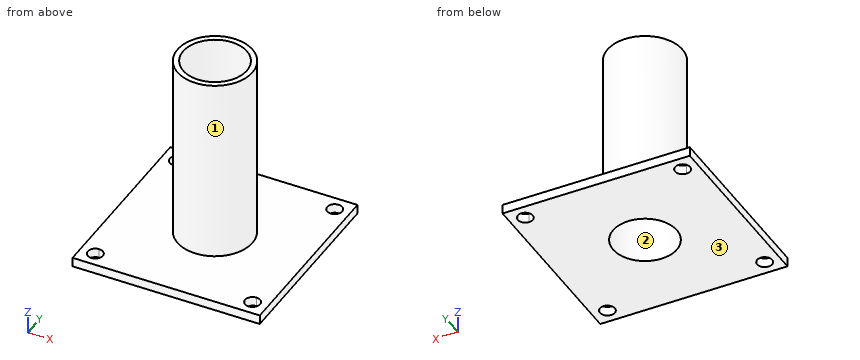
from build123d import *

# Parameters (mm, degrees)
F0_W     = 50
F0_H     = 50
F0_R     = 10
F0_R_2   = 8.5
F1_DEPTH = 2.5
F2_DEPTH = 25
F4_R     = 8.5
F4_R_2   = 2.5
F5_DEPTH = 2
F4_R_3   = 10
F6_DEPTH = 25
F7_R     = 2.5
F8_DEPTH = 25


with BuildPart() as f1:
    # F0 (on Top) → F1 (new body)
    with BuildSketch(Plane.XY):
        Rectangle(F0_W, F0_H)
        with BuildLine():
            ThreePointArc((-21, 19), (-22.414214, 22.414214), (-19, 21))
            Line((-19, 21), (19, 21))
            ThreePointArc((19, 21), (21, 23), (23, 21))
            ThreePointArc((23, 21), (22.414214, 19.585786), (21, 19))
            Line((21, 19), (21, -19))
            ThreePointArc((21, -19), (22.414214, -19.585786), (23, -21))
            ThreePointArc((23, -21), (21, -23), (19, -21))
            Line((19, -21), (-19, -21))
            ThreePointArc((-19, -21), (-22.414214, -22.414214), (-21, -19))
            Line((-21, -19), (-21, 19))
        make_face(mode=Mode.SUBTRACT)
        with BuildLine():
            Line((19, 21), (-19, 21))
            ThreePointArc((-19, 21), (-19.585786, 19.585786), (-21, 19))
            Line((-21, 19), (-21, -19))
            ThreePointArc((-21, -19), (-19.585786, -19.585786), (-19, -21))
            Line((-19, -21), (19, -21))
            ThreePointArc((19, -21), (19.585786, -19.585786), (21, -19))
            Line((21, -19), (21, 19))
            ThreePointArc((21, 19), (19.585786, 19.585786), (19, 21))
        make_face()
        Circle(F0_R, mode=Mode.SUBTRACT)
        Circle(F0_R)
        Circle(F0_R_2, mode=Mode.SUBTRACT)
    extrude(amount=-F1_DEPTH)

    # F0 (on Top) → F2 (join)
    with BuildSketch(Plane.XY):
        Circle(F0_R)
        Circle(F0_R_2, mode=Mode.SUBTRACT)
    extrude(amount=F2_DEPTH)

    # F4 (on offset) → F5 (join)
    with BuildSketch(Plane.XY.offset(25)):
        Circle(F4_R)
        Circle(F4_R_2, mode=Mode.SUBTRACT)
    extrude(amount=F5_DEPTH)

    # F4 (on offset) → F6 (join)
    with BuildSketch(Plane.XY.offset(25)):
        Circle(F4_R_3)
        Circle(F4_R, mode=Mode.SUBTRACT)
    extrude(amount=F6_DEPTH)

    # F7 (on Right) → F8 (cut)
    with BuildSketch(Plane.YZ):
        with Locations((0, 7.303349)):
            Circle(F7_R)
    extrude(amount=-F8_DEPTH, mode=Mode.SUBTRACT)


solid = f1.part
The listing builds one solid part. Answer for the finished solid, in the listing's coordinates (mm). Face numbers are marked on the shaded views. Coordinates: 2 decimals unless noted, no trailing zeros. Write each loop counter-clockwise with the first axis right and the second up, starting at its lowest first coordinate (ties: lowest second). Pieces come first, ordered by that corner, then holes. Notation, with made-up numbers: M 14.5,69.5 L 39.5,69.5 A14 cw 39.5,78.5 Z; hole C 36.25,34 d11. An arc over 180 degrees is marked long. Put each result on its own line as item: value. Start each with the question number.
1. Consider line 1 (X direction, y = 21, z = -1.4); line 2 (Y direction, x = 0, z = 39.5); line 3 (Z direction, x = 9, y = 14). Determine where each line is inside the solid, lowest interval first. Write a range as from..to.
2. A cutting plane is placed at B-B on z = 39. Write down the section's boundary in (x, y), then the cut area to 3 significant figures.
3. A cutting plane is placed at D-D on y = 16. Write down the section's boundary in (x, z).
4. A cutting plane is placed at A-A on y = 0. Write down the section's boundary in (x, z).
5. Flat-ended cylindrical pins translate along their axes: P1, Ø4.5, axis at x = -21, y = 21, coming from the +Z side; P2, Ø4.5, axis at y = 0, z = 7.3, coming from the -X side; P3, Ø12, axis at y = 17.5, z = 39, coming from the -X side; P4, Ø8, axis at y = 3, z = 26.5, coming from the +X side. Find the tip coordinate at first contact, or state that the pin passes through.
6. A cutting plane is placed at C-C on x = 3.5. Write down the section's boundary in (y, z).
7. For a pull along X with two mould halves and no side action, classify the marked faces 1, 2 and 3 as pulls with the +X half, pulls with the -X half, needs draft (parallel to the pull), parting line crosses it, or undercut.
Resolved:
1. line 1: x = -25..-23, -19..19, 23..25
1. line 2: y = -10..-8.5, 8.5..10
1. line 3: z = -2.5..0
2. outline: C 0,0 d20; hole C 0,0 d17
2. area: 87.2 mm2
3. outline: M -25,-2.5 L 25,-2.5 L 25,0 L -25,0 Z
4. outline: M -25,-2.5 L -8.5,-2.5 L -8.5,4.8 L -10,4.8 L -10,0 L -25,0 Z; M -10,9.8 L -8.5,9.8 L -8.5,25 L -2.5,25 L -2.5,27 L -8.5,27 L -8.5,50 L -10,50 Z; M 2.5,25 L 8.5,25 L 8.5,-2.5 L 25,-2.5 L 25,0 L 10,0 L 10,50 L 8.5,50 L 8.5,27 L 2.5,27 Z
5. P1: stops at z = 0
5. P2: stops at x = 8.2
5. P3: passes through
5. P4: stops at x = 10
6. outline: M -25,-2.5 L -7.75,-2.5 L -7.75,25 L 7.75,25 L 7.75,-2.5 L 25,-2.5 L 25,0 L 9.37,0 L 9.37,50 L 7.75,50 L 7.75,27 L -7.75,27 L -7.75,50 L -9.37,50 L -9.37,0 L -25,0 Z
7. face 1: parting line crosses it
7. face 2: undercut
7. face 3: needs draft
